Geometry: see drawing. Coordinates: mm, zero at the bounding-box minimum. Round coordinates to 2 decimals unless told otherwise and drop trailing zeros. Loops run counter-clockwise (first coordinate to the right, second up) from the corner with the lowest first, then second, coordinate; pieces in that order, holes last. Notation, with made-up numbers: (16, 34) - (49, 34) arc R14 ccw to (49, 47) - close; hole circle Ø9 at (53, -32). An arc over 180 degrees is marked (long way). Answer in a Markdown table with one row per item. Add a question column.
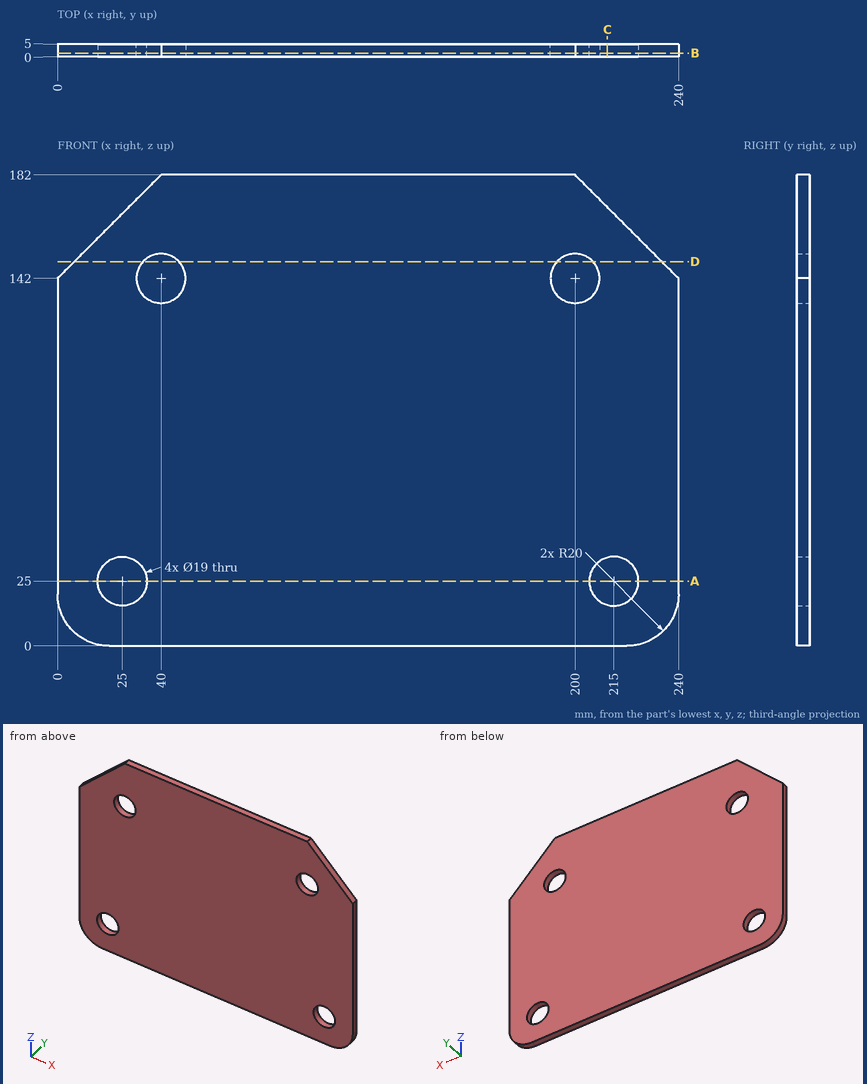
1) Contact query for a flat-ended pin moving along its axis: pin 1 Ø2 at (y, z) = (1.5, 111) entering from -X. Output: stop coordinate, or through.
2) Section A-A, the plane z = 25. Return the cut outline in (x, y).
3) Section B-B, the plane y = 1.5. Return the cut outline in (x, z).
4) Section D-D, the plane z = 148.5. Return the cut outline in (x, y), and give its area (3 significant figures).
5) Section C-C, the plane x = 212.5. Return the cut outline in (y, z), and give its area (3 significant figures).
6) Material intervals for line 1 along X through (y, z) = (1.1, 135); line 2 along X through (y, z) = (0.45, 144.5); line 3 along Z through (x, y) = (33, 2.15), sorted ascending. Write a range as from..to.
Evaluation:
| question | item | result |
|---|---|---|
| 1 | pin 1 | stops at x = 0 |
| 2 | outline | (0, 0) - (15.5, 0) - (15.5, 5) - (0, 5) - close; (34.5, 0) - (205.5, 0) - (205.5, 5) - (34.5, 5) - close; (224.5, 0) - (240, 0) - (240, 5) - (224.5, 5) - close |
| 3 | outline | (0, 20) arc R20 ccw to (20, 0) - (220, 0) arc R20 ccw to (240, 20) - (240, 142) - (200, 182) - (40, 182) - (0, 142) - close; hole circle Ø19 at (25, 25); hole circle Ø19 at (40, 142); hole circle Ø19 at (200, 142); hole circle Ø19 at (215, 25) |
| 4 | outline | (6.5, 0) - (33.07, 0) - (33.07, 5) - (6.5, 5) - close; (46.93, 0) - (193.07, 0) - (193.07, 5) - (46.93, 5) - close; (206.93, 0) - (233.5, 0) - (233.5, 5) - (206.93, 5) - close |
| 4 | area | 996 mm² |
| 5 | outline | (0, 0) - (5, 0) - (5, 15.83) - (0, 15.83) - close; (0, 34.17) - (5, 34.17) - (5, 169.5) - (0, 169.5) - close |
| 5 | area | 756 mm² |
| 6 | line 1 | x = 0..33.58, 46.42..193.58, 206.42..240 |
| 6 | line 2 | x = 2.5..30.83, 49.17..190.83, 209.17..237.5 |
| 6 | line 3 | z = 0..19.88, 30.12..135.58, 148.42..175 |
